```python
from build123d import *

# Parameters (mm, degrees)
SKETCH1_R           = 3
BOSS_EXTRUDE1_DEPTH = 10
SKETCH2_R           = 1.45
CUT_EXTRUDE1_DEPTH  = 142.244468918
BOSS_EXTRUDE2_DEPTH = 10
BOSS_EXTRUDE3_DEPTH = 10
SKETCH8_W           = 62.731065403
SKETCH8_H           = 467.056503757
CUT_EXTRUDE5_DEPTH  = 303.045371757


with BuildPart() as part:
    # Sketch1 → Boss-Extrude1 (new body)
    with BuildSketch(Plane.XY):
        with BuildLine():
            Line((-60, -125), (60, -125))
            ThreePointArc((60, -125), (63.535533906, -123.535533906), (65, -120))
            Line((65, -120), (65, 120))
            ThreePointArc((65, 120), (63.535533906, 123.535533906), (60, 125))
            Line((60, 125), (-60, 125))
            ThreePointArc((-60, 125), (-63.535533906, 123.535533906), (-65, 120))
            Line((-65, 120), (-65, -120))
            ThreePointArc((-65, -120), (-63.535533906, -123.535533906), (-60, -125))
        make_face()
        with Locations((-60, 120)):
            Circle(SKETCH1_R, mode=Mode.SUBTRACT)
        with Locations((60, 120)):
            Circle(SKETCH1_R, mode=Mode.SUBTRACT)
        with Locations((-60, -120)):
            Circle(SKETCH1_R, mode=Mode.SUBTRACT)
        with Locations((60, -120)):
            Circle(SKETCH1_R, mode=Mode.SUBTRACT)
        with BuildLine():
            Line((-50, -115), (50, -115))
            ThreePointArc((50, -115), (53.535533906, -113.535533906), (55, -110))
            Line((55, -110), (55, 110))
            ThreePointArc((55, 110), (53.535533906, 113.535533906), (50, 115))
            Line((50, 115), (-50, 115))
            ThreePointArc((-50, 115), (-53.535533906, 113.535533906), (-55, 110))
            Line((-55, 110), (-55, -110))
            ThreePointArc((-55, -110), (-53.535533906, -113.535533906), (-50, -115))
        make_face(mode=Mode.SUBTRACT)
    extrude(amount=BOSS_EXTRUDE1_DEPTH)

    # Sketch2 → Cut-Extrude1 (cut, through all)
    with BuildSketch(Plane(origin=(0, 0, 0), x_dir=(-1, 0, 0), z_dir=(0, 0, -1))):
        with Locations((-35, 120)):
            Circle(SKETCH2_R)
        with Locations((-60, 95)):
            Circle(SKETCH2_R)
        with Locations((-60, 25)):
            Circle(SKETCH2_R)
        with Locations(Location((-60, -25, 0), (0, 0, 180))):
            Circle(SKETCH2_R)
        with Locations(Location((-60, -95, 0), (0, 0, 180))):
            Circle(SKETCH2_R)
        with Locations(Location((-35, -120, 0), (0, 0, 180))):
            Circle(SKETCH2_R)
        with Locations((35, -120)):
            Circle(SKETCH2_R)
        with Locations((60, -95)):
            Circle(SKETCH2_R)
        with Locations((60, -25)):
            Circle(SKETCH2_R)
        with Locations(Location((60, 25, 0), (0, 0, 180))):
            Circle(SKETCH2_R)
        with Locations(Location((60, 95, 0), (0, 0, 180))):
            Circle(SKETCH2_R)
        with Locations(Location((35, 120, 0), (0, 0, 180))):
            Circle(SKETCH2_R)
    extrude(amount=-CUT_EXTRUDE1_DEPTH, mode=Mode.SUBTRACT)

    # Sketch3 → Boss-Extrude2 (add, through all)
    with BuildSketch(Plane.XY.offset(10)):
        with BuildLine():
            Line((-20, -214.79), (-20, -130))
            ThreePointArc((-20, -130), (-21.464466094, -126.464466094), (-25, -125))
            Line((-25, -125), (25, -125))
            ThreePointArc((25, -125), (21.464466094, -126.464466094), (20, -130))
            Line((20, -130), (20, -214.79))
            ThreePointArc((20, -214.79), (0, -234.79), (-20, -214.79))
        make_face()
    extrude(amount=-BOSS_EXTRUDE2_DEPTH)

    # Sketch5 → Boss-Extrude3 (add)
    with BuildSketch(Plane.XY.offset(10)):
        with BuildLine():
            ThreePointArc((-38.890872965, 126.464466094), (-40.512989709, 125.380602337), (-42.426406871, 125))
            Line((-42.426406871, 125), (42.426406871, 125))
            ThreePointArc((42.426406871, 125), (37.807009209, 128.086582838), (38.890872965, 133.535533906))
            Line((38.890872965, 133.535533906), (67.855339059, 162.5))
            Line((67.855339059, 162.5), (102.25, 162.5))
            ThreePointArc((102.25, 162.5), (124.75, 185), (102.25, 207.5))
            Line((102.25, 207.5), (42.144660941, 207.5))
            Line((42.144660941, 207.5), (-38.890872965, 126.464466094))
        make_face()
    extrude(amount=-BOSS_EXTRUDE3_DEPTH)

    # Sketch8 → Cut-Extrude5 (cut, through all)
    with BuildSketch(Plane.ZY.offset(65)):
        with Locations((34.365532702, -16.017183146)):
            Rectangle(SKETCH8_W, SKETCH8_H)
    extrude(amount=-CUT_EXTRUDE5_DEPTH, mode=Mode.SUBTRACT)


solid = part.part
```
Work out the finished part from the listing and answer in its coordinate system (mm). Give positions to 0.01 mm unless a question says otherwise; leave off trailing zeros. Write each loop counter-clockwise with the first axis right and the second up, starting at its lowest first coordinate (ties: lowest second). Pieces come first, ordered by that corner, then holes. Notation, with made-up numbers: (-20, 51.25) - (13, 51.25) arc R20 ccw to (13, 68.25) - close; hole circle Ø3 at (55, -0.5). An arc over 180 degrees is marked (long way). Use one line per item in the form item = value.
1. A cutting plane is placed at C-C (z = 0.65). State how many separate pieces and enclosed holes the cut face has, and give its area (3 significant figures).
Filled in:
separate_pieces = 1
enclosed_holes = 17
area = 18,400 mm^2
2. Determine the mould class of faces 1 (the face through (53.17, 147.815, 1.521)), 2 (the face through (2.194, 167.549, 1.521)), 3 (the face through (58, 18, 3)) for opening direction Y: released by +Y, released by -Y, zero draft, split by the parting line, or undercut.
Filled in:
face_1 = undercut
face_2 = released by +Y
face_3 = zero draft
3. A cutting plane is placed at B-B (x = -5). Write down the section's boundary in (y, z), and give its area (3 significant figures).
Filled in:
outline = (-234.15, 0) - (-115, 0) - (-115, 3) - (-234.15, 3) - close; (115, 0) - (160.36, 0) - (160.36, 3) - (115, 3) - close
area = 494 mm^2
4. Consider L1, parallel to X at y = -120, z = 1.7; L2, parallel to X at y = 95, z = 1.9; L3, parallel to X at y = 12, z = 2.55. Determine where each line is inside the solid, lowest interval first.
Filled in:
L1 = -65 to -63, -57 to -36.45, -33.55 to 33.55, 36.45 to 57, 63 to 65
L2 = -65 to -61.45, -58.55 to -55, 55 to 58.55, 61.45 to 65
L3 = -65 to -55, 55 to 65
5. Each of these flat-tipped pins is pushed along its axis until it touches: pin 1 Ø1.5 at (x, z) = (86, 1.5) entering from -Y; pin 2 Ø1.5 at (x, z) = (-1.5, 1.5) entering from -Y; pin 3 Ø1.5 at (x, z) = (19.5, 1) entering from +Y. Where does it stop, or does it pass through?
Filled in:
pin_1 = 162.5
pin_2 = -234.78
pin_3 = 185.61
6. A cutting plane is placed at A-A (y = -63.5). Write down the section's boundary in (x, z), and give its area (3 significant figures).
Filled in:
outline = (-65, 0) - (-55, 0) - (-55, 3) - (-65, 3) - close; (55, 0) - (65, 0) - (65, 3) - (55, 3) - close
area = 60.0 mm^2
7. A cutting plane is placed at D-D (y = 150.5). Write down the section's boundary in (x, z).
Filled in:
outline = (-14.86, 0) - (55.86, 0) - (55.86, 3) - (-14.86, 3) - close
